Input: dimensioned drawing with shaded views. Units: mm. Origin: part minimum x, y, z. A direction names the side the tool comes from. Coordinates: 2 decimals unless noted, no trailing zeros. Order: outer loops, then holes, each group sorted by start corner. A loop starts at its lowest first (then second) coordinate and runs counter-clockwise, first axis right, second up. Notation, with made-up numbers: (20, 66.5) -> (46, 66.5) arc R16 ccw to (46, 82.5) -> close; hole circle Ø1 at (67.5, 22). An arc over 180 degrees is marked (long way). Answer in a Markdown table with one row per item. Add a question column.
1) Pull-direction query (Y, two-part tool) for the marked faces 3, 4 and 5; classes: +Y half, -Y half, draft (parallel to the pull), parting line (faces both ways), or undercut.
2) Set-up query: the marked faces 1 and 2. Return all of +Z, -Z, +X, -X, +Y, -Y with unobstructed straight access to the full face (end or side cutting, diameter ignored); none if empty.
3) Contact query for flat-ended pins moving along their axis: P1, Ø1, axis at y = 8, z = 0.5, coming from the -X side; P2, Ø3, axis at x = 5.5, y = 6, coming from the +Z side; P3, Ø5, axis at x = 8, y = 4, coming from the +Z side; P4, Ø2, axis at y = 8, z = 2, coming from the +X side. Output: stop coordinate, or through.
4) Section query C-C on z = 3. Return the cut outline in (x, y).
5) Section query A-A on x = 6. Return the cut outline in (y, z).
6) Ray query, line 1 (X direction, y = 6, z = 1.55); line 2 (Y direction, x = 6, z = 2.55). Return the intervals inside material, ascending. Write a range as from..to.
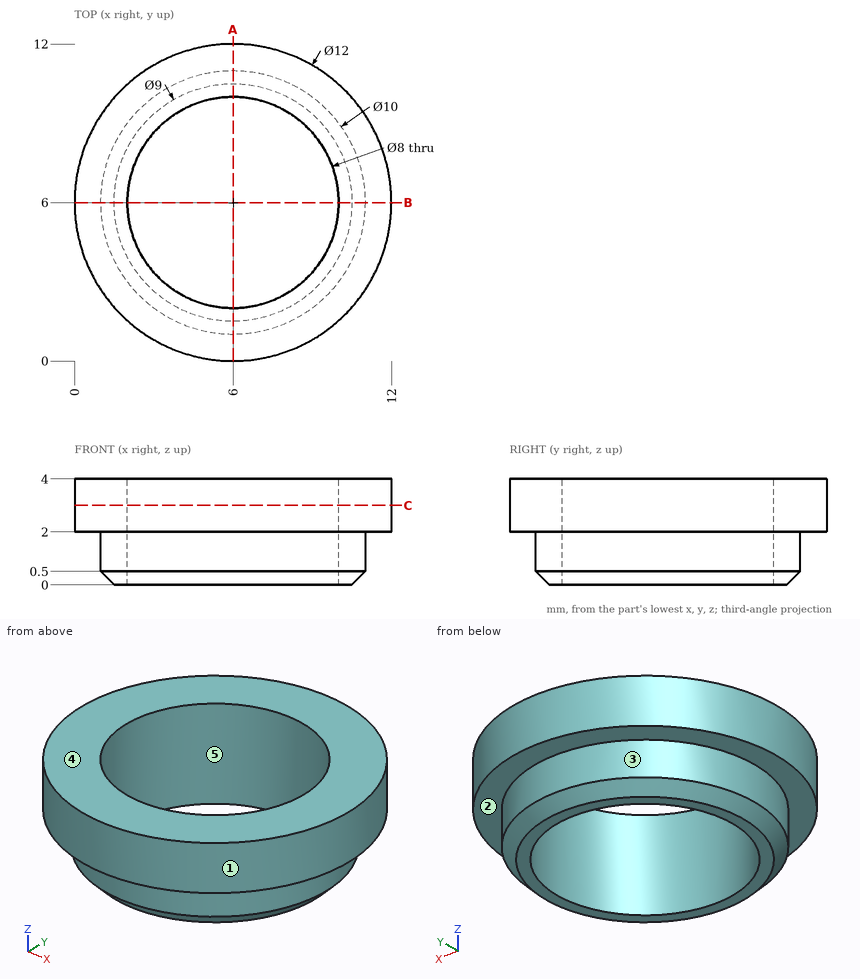
Result:
| question | item | result |
|---|---|---|
| 1 | face 3 | parting line |
| 1 | face 4 | draft |
| 1 | face 5 | undercut |
| 2 | face 1 | +Z, -Z |
| 2 | face 2 | -Z |
| 3 | P1 | x = 1.23 |
| 3 | P2 | through |
| 3 | P3 | z = 4 |
| 3 | P4 | x = 11.92 |
| 4 | outline | circle Ø12 at (6, 6); hole circle Ø8 at (6, 6) |
| 5 | outline | (0, 2) -> (1, 2) -> (1, 0.5) -> (1.5, 0) -> (2, 0) -> (2, 4) -> (0, 4) -> close; (10, 0) -> (10.5, 0) -> (11, 0.5) -> (11, 2) -> (12, 2) -> (12, 4) -> (10, 4) -> close |
| 6 | line 1 | 1..2, 10..11 |
| 6 | line 2 | 0..2, 10..12 |
